```python
from build123d import *

# Parameters (mm, degrees)
BOSS_EXTRUDE1_DEPTH             = 10
TAP_DRILL_FOR_M4X0_7_TAP1_D     = 3.3
TAP_DRILL_FOR_M4X0_7_TAP1_DEPTH = 5
TAP_DRILL_FOR_M4X0_7_TAP1_TIP   = 0.991420021
TAP_DRILL_FOR_M5X0_8_TAP3_D     = 4.2
TAP_DRILL_FOR_M5X0_8_TAP2_D     = 4.2
TAP_DRILL_FOR_M5X0_8_TAP2_DEPTH = 7
TAP_DRILL_FOR_M5X0_8_TAP2_TIP   = 1.2618073
FILLET1_R                       = 1


with BuildPart() as part:
    # Sketch1 → Boss-Extrude1 (new body)
    with BuildSketch(Plane.XY):
        Polygon((15, 40), (-74.5, 40), (-74.5, 0), (74.5, 0), (74.5, 40), (55, 40), (55, 19.855), (38.005, 19.855), (38.005, 16.85), (31.995, 16.85), (31.995, 19.855), (15, 19.855), align=None)
    extrude(amount=-BOSS_EXTRUDE1_DEPTH)

    # Tap Drill for M4x0.7 Tap1
    with Locations(Plane(origin=(25, 19.855, -5), x_dir=(1, 0, 0), z_dir=(0, 1, 0))):
        with Locations((0, 0), (20, 0)):
            Hole(TAP_DRILL_FOR_M4X0_7_TAP1_D / 2, depth=TAP_DRILL_FOR_M4X0_7_TAP1_DEPTH)
            with Locations((0, 0, -(TAP_DRILL_FOR_M4X0_7_TAP1_DEPTH + TAP_DRILL_FOR_M4X0_7_TAP1_TIP / 2))):  # 118° drill point
                Cone(0, TAP_DRILL_FOR_M4X0_7_TAP1_D / 2, TAP_DRILL_FOR_M4X0_7_TAP1_TIP, mode=Mode.SUBTRACT)

    # Tap Drill for M5x0.8 Tap3 (through all)
    with Locations(Plane(origin=(-65, 30, 0), x_dir=(1, 0, 0), z_dir=(0, 0, 1))):
        with Locations((0, 0), (0, -20), (130, -20), (130, 0)):
            Hole(TAP_DRILL_FOR_M5X0_8_TAP3_D / 2)

    # Tap Drill for M5x0.8 Tap2
    with Locations(Plane(origin=(-60, 0, -5), x_dir=(-1, 0, 0), z_dir=(0, -1, 0))):
        with Locations((0, 0), (-60, 0), (-120, 0)):
            Hole(TAP_DRILL_FOR_M5X0_8_TAP2_D / 2, depth=TAP_DRILL_FOR_M5X0_8_TAP2_DEPTH)
            with Locations((0, 0, -(TAP_DRILL_FOR_M5X0_8_TAP2_DEPTH + TAP_DRILL_FOR_M5X0_8_TAP2_TIP / 2))):  # 118° drill point
                Cone(0, TAP_DRILL_FOR_M5X0_8_TAP2_D / 2, TAP_DRILL_FOR_M5X0_8_TAP2_TIP, mode=Mode.SUBTRACT)

    # Fillet1
    fillet1_edges = [part.edges().sort_by_distance(p)[0] for p in [
        (55, 40, -5),
        (15, 40, -5),
    ]]
    fillet(fillet1_edges, radius=FILLET1_R)


solid = part.part
```
Read the model definition and answer for the solid it produces. Units are mm, in the model's axes. A direction names the side the tool comes from. Round coordinates to 2 decimals unless told otherwise and drop trailing zeros. Write each loop counter-clockwise with the first axis right and the second up, starting at its lowest first coordinate (ties: lowest second). Pieces come first, ordered by that corner, then holes. Notation, with made-up numbers: (-12, 58.25) -> (18, 58.25) arc R14 cw to (18, 63.25) -> close; hole circle Ø10 at (-28.75, -34). An arc over 180 degrees is marked (long way). Answer in a Markdown table with one row per item. Add a question column.
1) Find section B-B, the plane x = -65. Determine the outline of the cut face in (y, z), and give its area (3 significant figures).
2) Given P1, Ø2, axis at x = 22, z = -8.5, coming from the +Y side (3 decimals); P2, Ø3, axis at x = 45, z = -5, coming from the +Y side; P3, Ø2.5, axis at x = -65, y = 30, coming from the +Z side (3 decimals); P4, Ø4, axis at x = 60, z = -5, coming from the -Y side, each flat-ended and moving along its own axis, determine where each tip first touches the part or whether it passes through.
3) Find section D-D, the plane y = 4. Determine the outline of the cut face in (x, z), and give its area (3 significant figures).
4) Consider line 1 (X direction, y = 17, z = -5) (3 decimals); line 2 (X direction, y = 23.5, z = -4.5); line 3 (Y direction, x = 65, z = -6.5). Determine where each line is inside the solid, lowest interval first.
5) Which of the six approach directions +Z, -Z, +X, -X, +Y, -Y give full straight-line access (tool end or side, diameter ignored) to faces 1 (the face through (26.65, 17.32, -5.07)), 2 (the face through (62.003, 3.549, -5.631)), 3 (the face through (55, 30, -5))?
6) Find section A-A, the plane y = 10. Determine the outline of the cut face in (x, z).
7) Find section C-C, the plane y = 26. Determine the outline of the cut face in (x, z), and give its area (3 significant figures).
8) Determine the mould class of faces 4 (the face through (-74.5, 20, -5)), 5 (the face through (-1, 0, -2.7)), 6 (the face through (64.031, 28.137, -5.07)) for opening direction X: pulls with the +X half, pulls with the -X half, needs draft (parallel to the pull), parting line crosses it, or undercut.
Findings below:
| question | item | result |
|---|---|---|
| 1 | outline | (0, -10) -> (7.9, -10) -> (7.9, 0) -> (0, 0) -> close; (12.1, -10) -> (27.9, -10) -> (27.9, 0) -> (12.1, 0) -> close; (32.1, -10) -> (40, -10) -> (40, 0) -> (32.1, 0) -> close |
| 1 | area | 316 mm² |
| 2 | P1 | y = 19.855 |
| 2 | P2 | y = 14.76 |
| 2 | P3 | through |
| 2 | P4 | y = 7.06 |
| 3 | outline | (-74.5, -10) -> (74.5, -10) -> (74.5, 0) -> (-74.5, 0) -> close; hole circle Ø4.2 at (-60, -5); hole circle Ø4.2 at (0, -5); hole circle Ø4.2 at (60, -5) |
| 3 | area | 1,450 mm² |
| 4 | line 1 | -74.5 to 23.35, 26.65 to 31.995, 38.005 to 43.35, 46.65 to 74.5 |
| 4 | line 2 | -74.5 to 15, 55 to 74.5 |
| 4 | line 3 | 0 to 7.9, 12.1 to 27.9, 32.1 to 40 |
| 5 | face 1 | +Y |
| 5 | face 2 | -Y |
| 5 | face 3 | +Z, -Z, +Y |
| 6 | outline | (-74.5, -10) -> (-67.1, -10) -> (-67.1, 0) -> (-74.5, 0) -> close; (-62.9, -10) -> (62.9, -10) -> (62.9, 0) -> (-62.9, 0) -> close; (67.1, -10) -> (74.5, -10) -> (74.5, 0) -> (67.1, 0) -> close |
| 7 | outline | (-74.5, -10) -> (15, -10) -> (15, 0) -> (-74.5, 0) -> close; (55, -10) -> (74.5, -10) -> (74.5, 0) -> (55, 0) -> close |
| 7 | area | 1,090 mm² |
| 8 | face 4 | pulls with the -X half |
| 8 | face 5 | needs draft |
| 8 | face 6 | undercut |
